from build123d import *

# Parameters (mm, degrees)
F0_W           = 39
F0_H           = 19
F1_DEPTH       = 20
F2_D           = 5.5
F2_DEPTH       = 20
F2_CBORE_D     = 9.75
F2_CBORE_DEPTH = 5
F2_TIP         = 1.6523667023
F3_D           = 4.2
F3_DEPTH       = 22.4
F3_TIP         = 1.2618073


with BuildPart() as f1:
    # F0 (on Top) → F1 (new body)
    with BuildSketch(Plane.XY):
        Rectangle(F0_W, F0_H)
    extrude(amount=-F1_DEPTH)

    # F2
    with Locations(Plane.XY):
        with Locations((-9.5, 0)):
            CounterBoreHole(F2_D / 2, F2_CBORE_D / 2, F2_CBORE_DEPTH, depth=F2_DEPTH)
            with Locations((0, 0, -(F2_DEPTH + F2_TIP / 2))):  # 118° drill point
                Cone(0, F2_D / 2, F2_TIP, mode=Mode.SUBTRACT)

    # F3
    with Locations(Plane.XY):
        with Locations((9.5, 0)):
            Hole(F3_D / 2, depth=F3_DEPTH)
            with Locations((0, 0, -(F3_DEPTH + F3_TIP / 2))):  # 118° drill point
                Cone(0, F3_D / 2, F3_TIP, mode=Mode.SUBTRACT)


solid = f1.part
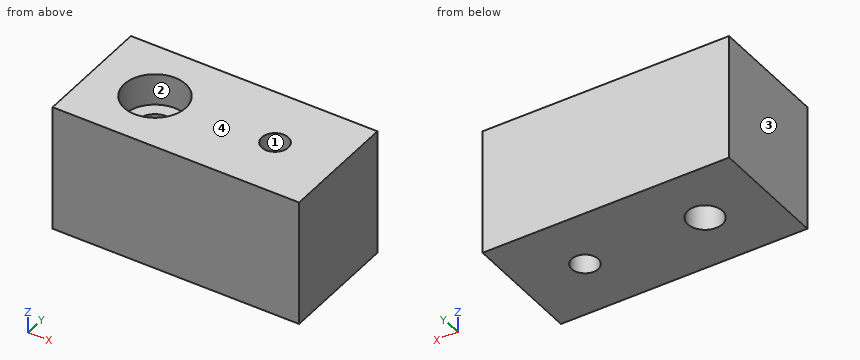
Can you work these out from the model? Positions are in its coordinate system, mm. Face numbers are marked on the shaded views. Give positions to 0.01 mm unless a question says otherwise; leave off trailing zeros. Order: outer loops, then holes, each group sorted by start corner. A loop starts at its lowest first (then second) coordinate and runs counter-clockwise, first axis right, second up. Notation, with made-up numbers: M 60.5,13 L 102.5,13 A29 ccw 102.5,36 Z; hole C 78.25,89.25 d10. An arc over 180 degrees is marked long. Use one line per item in the form item = value. Start each with the question number.
Item 1: If I drill on line 1 along X through (y, z) = (1.5, -14); line 2 along Y through (x, z) = (-9.5, -3.05) (3 decimals); line 3 along Y through (x, z) = (-9.5, -10), over which ranges is the centre line in solid material (lowest first)?
Item 2: Will this pin go through, and if not, where does the flat tip stop? pin 1 Ø3 at (x, y) = (-8, -2.5) entering from +Z.
Item 3: If we section it at D-D (x = 9.5): Write out the boundary of the cut face in (y, z), then the cut area to 3 significant figures.
Item 4: If we section it at A-A (x = -9.5): Write out the boundary of the cut face in (y, z) (3 decimals), then the cut area to 3 significant figures.
Item 5: If we section it at C-C (z = -15.75): Write out the boundary of the cut face in (x, y), then the cut area to 3 significant figures.
Item 6: If we section it at B-B (y = 0): Write out the boundary of the cut face in (x, z) (3 decimals).
Item 7: We'd pull the mould along X, two halves only. Please class the marked faces 1, 2, 3 and 4: +X half, -X half, draft (parallel to the pull), parting line (faces both ways), or undercut.
Outcome:
q1.line_1 = -19.5 to -11.8, -7.2 to 8.03, 10.97 to 19.5
q1.line_2 = -9.5 to -4.875, 4.875 to 9.5
q1.line_3 = -9.5 to -2.75, 2.75 to 9.5
q2.pin_1 = -5
q3.outline = M -9.5,-20 L -2.1,-20 L -2.1,0 L -9.5,0 Z; M 2.1,-20 L 9.5,-20 L 9.5,0 L 2.1,0 Z
q3.area = 296 mm2
q4.outline = M -9.5,-20 L -2.75,-20 L -2.75,-5 L -4.875,-5 L -4.875,0 L -9.5,0 Z; M 2.75,-20 L 9.5,-20 L 9.5,0 L 4.875,0 L 4.875,-5 L 2.75,-5 Z
q4.area = 249 mm2
q5.outline = M -19.5,-9.5 L 19.5,-9.5 L 19.5,9.5 L -19.5,9.5 Z; hole C -9.5,0 d5.5; hole C 9.5,0 d4.2
q5.area = 703 mm2
q6.outline = M -19.5,-20 L -12.25,-20 L -12.25,-5 L -14.375,-5 L -14.375,0 L -19.5,0 Z; M -6.75,-20 L 7.4,-20 L 7.4,0 L -4.625,0 L -4.625,-5 L -6.75,-5 Z; M 11.6,-20 L 19.5,-20 L 19.5,0 L 11.6,0 Z
q7.face_1 = undercut
q7.face_2 = undercut
q7.face_3 = -X half
q7.face_4 = draft
